Here's the drawing with two shaded views (mm, measured from the low corner). I have some questions. A direction names the side the tool comes from. Round coordinates to 2 decimals unless told otherwise and drop trailing zeros. Order: outer loops, then holes, each group sorted by start corner. A loop starts at its lowest first (then second) coordinate and runs counter-clockwise, first axis right, second up.
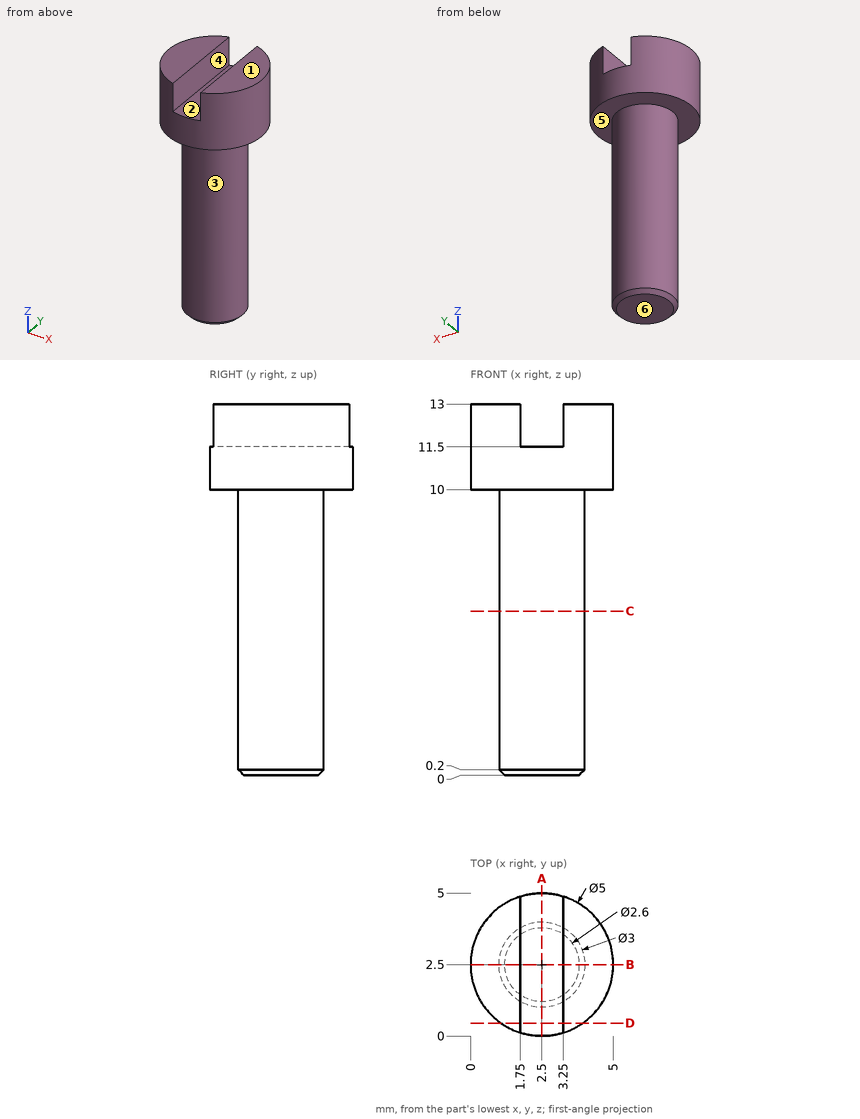
1. I need wall thicknesses on probe 1 along Z at (x, y) = (3, 1.8); probe 2 along Z at (x, y) = (1.6, 0.5); probe 3 along Y at (x, z) = (2.4, 11). Which ranges of each line are inside material? Lowest first, please.
Evaluation:
probe 1: z = 0 to 11.5
probe 2: z = 10 to 13
probe 3: y = 0 to 5
2. On a 3-axis mill with a long thin cutter (end or side, diameter ignored), from which of +Z, -Z, +X, -X, +Y, -Y can I reach the whole of each face in a straight line? I mean the marked faces 5 and 6. Say none if no direction works.
Evaluation:
face 5: -Z
face 6: -Z, +X, -X, +Y, -Y
3. If we section it at D-D, the plane y = 0.45: Write out the boundary of the cut face in (x, z), and give its area (3 significant figures).
Evaluation:
outline: (1.07, 10) - (3.93, 10) - (3.93, 13) - (3.25, 13) - (3.25, 11.5) - (1.75, 11.5) - (1.75, 13) - (1.07, 13) - close
area: 6.34 mm2
4. If we mould it in two halves opening along X, with no side actions, what happens to the marked faces 1, 2, 3 and 4? For each: released by +X, released by -X, zero draft, split by the parting line, or undercut.
Evaluation:
face 1: zero draft
face 2: undercut
face 3: split by the parting line
face 4: undercut
5. If we section it at A-A, the plane x = 2.5: Write out the boundary of the cut face in (y, z), and give its area (3 significant figures).
Evaluation:
outline: (0, 10) - (1, 10) - (1, 0.2) - (1.2, 0) - (3.8, 0) - (4, 0.2) - (4, 10) - (5, 10) - (5, 11.5) - (0, 11.5) - close
area: 37.5 mm2
6. If we section it at C-C, the plane z = 5.75: Write out the boundary of the cut face in (x, y), and give its area (3 significant figures).
Evaluation:
outline: circle Ø3 at (2.5, 2.5)
area: 7.07 mm2
7. I'm going to push flat-ended pins straight in: P1, Ø1.6, axis at y = 1.5, z = 12.5, coming from the -X side; P2, Ø1.2, axis at x = 2.5, y = 2.5, coming from the +Z side; P3, Ø1.2, axis at y = 3.5, z = 12, coming from the +X side. Where does each tip first touch, or does it pass through?
Evaluation:
P1: stops at x = 0.01
P2: stops at z = 11.5
P3: stops at x = 4.97
8. If we section it at B-B, the plane y = 2.5: Write out the boundary of the cut face in (x, z).
Evaluation:
outline: (0, 10) - (1, 10) - (1, 0.2) - (1.2, 0) - (3.8, 0) - (4, 0.2) - (4, 10) - (5, 10) - (5, 13) - (3.25, 13) - (3.25, 11.5) - (1.75, 11.5) - (1.75, 13) - (0, 13) - close
